Autodesk Inventor part; units mm, degrees
ref_plane "YZ Plane" through (0, 0, 0) normal (1, 0, 0) x (0, 1, 0)
ref_plane "XZ Plane" through (0, 0, 0) normal (0, 1, 0) x (-1, 0, 0)
ref_plane "XY Plane" through (0, 0, 0) normal (0, 0, 1) x (1, 0, 0)
sketch "Sketch1" plane through (0, 0, 0) normal (0, 1, 0) x (-1, 0, 0)
  line L0 (-2, 6.5) -> (2, 6.5)
  line L1 (2, 6.5) -> (2, -6.5)
  line L2 (2, -6.5) -> (-2, -6.5)
  line L3 (-2, -6.5) -> (-2, 6.5)
  line L4 (-2, 6.5) -> (2, -6.5) construction
  line L5 (2, 6.5) -> (-2, -6.5) construction
  point P0 (0, 0)
  dimension "d0" = 4
  dimension "d1" = 13
extrude "Extrusion1" add sketch "Sketch1" along normal blind 4
sketch "Sketch2" plane through (2, 0, 6.5) normal (1, 0, 0) x (0, 0, -1)
  line L0 (0, 0) -> (0, 4)
  line L1 (0, 2) -> (13, 2) construction
  line L2 (13, 0) -> (13, 4)
  line L3 (2, 0) -> (11, 0)
  line L4 (11, 4) -> (2, 4)
  arc A0 (2, 4) -> (2, 0) centre (2, 2) ccw
  arc A1 (11, 0) -> (11, 4) centre (11, 2) ccw
  line L5 (0, 4) -> (13, 4)
  line L6 (0, 0) -> (13, 0)
  point P0 (6.5, 0)
  point P1 (6.5, 2)
extrude "Extrusion2" cut sketch "Sketch2" against normal blind 2 contours L0 A0 L6 | L0 L5 A0 | A1 L2 L6 | L5 L2 A1
sketch "Sketch3" plane through (-2, 0, -6.5) normal (-1, 0, 0) x (0, 0, 1)
  arc A0 (2, 4) -> (0, 2) centre (2, 2) ccw
  line L0 (0, 0) -> (0, 4)
  line L1 (0, 4) -> (13, 4)
  arc A1 (0, 2) -> (2, 0) centre (2, 2) ccw
  arc A2 (2, 4) -> (2, 0) centre (2, 2) ccw
  line L2 (11, 4) -> (2, 4)
  arc A3 (11, 0) -> (11, 4) centre (11, 2) ccw
  line L3 (11, 0) -> (2, 0)
  line L4 (13, 0) -> (13, 4)
  line L5 (0, 0) -> (13, 0)
  point P0 (6.5, 0)
  point P1 (13, 2)
extrude "Extrusion3" cut sketch "Sketch3" against normal blind 1 contours A0 L0 L1 | A1 L5 L0 | L1 L4 A3 | L4 L5 A3
sketch "Sketch4" plane through (-2, 0, -4.5) normal (-1, 0, 0) x (0, 0, 1)
  arc A0 (0, 4) -> (-2, 2) centre (0, 2) ccw
  circle A1 centre (0, 2) radius 1.5
  arc A2 (11, 2) -> (9, 4) centre (9, 2) ccw
  circle A3 centre (9, 2) radius 1.5
  point P0 (4.5, 0)
  dimension "d8" = 3
  dimension "d9" = 3
mark "Mark1"
sketch "Sketch5" plane through (-2, 0, -4.5) normal (-1, 0, 0) x (0, 0, 1)
  circle A0 centre (3, 2) radius 1
  circle A1 centre (0, 2) radius 1.5
  circle A2 centre (9, 2) radius 1.5
  line L0 (0, 4) -> (9, 4)
  circle A3 centre (6, 2) radius 1
  point P0 (4.5, 0)
  dimension "d10" = 2
  dimension "d11" = 3
  dimension "d12" = 9
  dimension "d15" = 3
mark "Mark2"
sketch "Sketch6" plane through (-2, 2, -1.5) normal (-1, 0, 0) x (0, 0, 1)
  circle A0 centre (0, 0) radius 1
  circle A1 centre (0, 0) radius 0.5
  circle A2 centre (3, 0) radius 1
  circle A3 centre (3, 0) radius 0.5
  point P0 (1.5, -2)
  dimension "d20" = 1
  dimension "d21" = 1
extrude "Extrusion4" add sketch "Sketch6" along normal blind 2 contours A1 | A3
sketch "Sketch7" plane through (2, 0, 4.5) normal (1, 0, 0) x (0, 0, -1)
  circle A0 centre (0, 2) radius 1.5
  circle A1 centre (9, 2) radius 1.5
  point P0 (4.5, 0)
mark "Mark3"
sketch "Sketch8" plane through (2, 0, 4.5) normal (1, 0, 0) x (0, 0, -1)
  circle A0 centre (6, 2) radius 1
  circle A1 centre (3, 2) radius 1
  circle A2 centre (3, 2) radius 0.75
  circle A3 centre (6, 2) radius 0.75
  point P0 (4.5, 0)
  dimension "d24" = 1.5
  dimension "d25" = 1.5
mark "Mark4"
sketch "Sketch11" plane through (0, 0, 6.5) normal (1, 0, 0) x (0, 0, -1)
  line L0 (-2.865, 2) -> (15.865, 2) construction
  line L1 (-0.865, 0) -> (13.865, 0)
  line L2 (13.865, 4) -> (-0.865, 4)
  arc A0 (-0.865, 4) -> (-0.865, 0) centre (-0.865, 2) ccw
  arc A1 (13.865, 0) -> (13.865, 4) centre (13.865, 2) ccw
  line L3 (2, 0) -> (11, 0)
  point P0 (6.5, 0)
  point P1 (6.5, 2)
  point P2 (6.5, 4)
  point P3 (6.5, 0)
  dimension "d31" = 18.73
extrude "Extrusion7" add sketch "Sketch11" against normal blind 1
sketch "Sketch12" plane through (0, 0, 6.5) normal (1, 0, 0) x (0, 0, -1)
  arc A0 (-0.865, 4) -> (-0.865, 0) centre (-0.865, 2) ccw
  circle A1 centre (-1.6, 2) radius 0.75
  circle A2 centre (2, 2) radius 1.5
  point P0 (6.5, 0)
  dimension "d34" = 1.5
  dimension "d35" = 3.6
extrude "Extrusion8" cut sketch "Sketch12" against normal blind 1 contours A1
mirror "Mirror1" about plane through (0, 0, 0) normal (0, 0, 1) of "Extrusion8"
equation "\"d9\" = d8"
equation "\"d11\" = 0.333333 * d12"
equation "\"d15\" = d11"
equation "\"d21\" = d20"
equation "\"d25\" = d24"
properties part number "2_pin_ear_female"
Check sheet for the modelled part. Datum: model origin and axes. Units: mm. A direction names the side the tool comes from. Coordinates: 2 decimals unless noted, no trailing zeros. Order: outer loops, then holes, each group sorted by start corner. A loop starts at its lowest first (then second) coordinate and runs counter-clockwise, first axis right, second up. Notation, with made-up numbers: M 40,11.25 L 86,11.25 A28 cw 86,42.25 Z; hole C -20,-7 d11. An arc over 180 degrees is marked long. One line per question, with ' | ' between items. Start each with the question number.
Item 1: Sectioned sample at D-D on x = -3.5. Record the cut outline in (y, z), and give its area (3 significant figures).
Item 2: Access from +Z, -Z, +X, -X, +Y, -Y to the whole of each face (thin tool, end or side, straight path). Record for faces 5 (the cylindrical face through (-1.5, 2, -6.5)), 6 (the cylindrical face through (-1.5, 2, 6.5)), 7 (the cylindrical face through (1, 2, 6.5)), 8 (the cylindrical face through (-3, 2, 1)), 9 (the cylindrical face through (1, 2, -6.5)).
Item 3: Sectioned sample at A-A on y = 2. Record the cut outline in (x, z) (3 decimals).
Item 4: Mould release check, pull along Y, two halves, no side actions. Record for faces 1 (the cylindrical face through (-0.493, 2.225, 7.385)), 2 (the flat face through (2, 2, 0)), 3 (the flat face through (0, 4, 0)), 4 (the cylindrical face through (-0.493, 1.956, -9.365)): pulls with the +Y half, pulls with the -Y half, needs draft (parallel to the pull), parting line crosses it, or undercut.
Item 5: Material ranges on line 1 (X direction, y = 3.25, z = -3.75); line 2 (Y direction, x = -0.5, z = 8.1); line 3 (Z direction, x = -2.8, y = 1.75), recorded low to high.
Item 6: Gauge pin test, flat ends, axial feed: P1, Ø2, axis at y = 2.5, z = -7, coming from the -X side; P2, Ø1.5, axis at x = 1, y = 1, coming from the -Z side; P3, Ø2, axis at y = 2, z = 8.1, coming from the -X side; P4, Ø0.9, axis at y = 2, z = -8.1, coming from the -X side. Record the tip position at first contact, or that the pin passes through.
Item 7: Sectioned sample at C-C on z = 1.5. Record the cut outline in (x, y).
Item 8: Sectioned sample at B-B on z = -8. Record the cut outline in (x, y), and give its area (3 significant figures).
Answer below:
1) outline: C 2,-1.5 d1; C 2,1.5 d1 | area: 1.57 mm^2
2) face 5: -Z, -X | face 6: +Z, -X | face 7: +Z, +X | face 8: -X | face 9: -Z, +X
3) outline: M -4,-2 L -2,-2 L -2,-6.5 L -1,-6.5 L -1,-7.35 L 0,-7.35 L 0,-6.5 L 2,-6.5 L 2,6.5 L 0,6.5 L 0,7.35 L -1,7.35 L -1,6.5 L -2,6.5 L -2,2 L -4,2 L -4,1 L -2,1 L -2,-1 L -4,-1 Z; M -1,-9.365 L 0,-9.365 L 0,-8.85 L -1,-8.85 Z; M -1,8.85 L 0,8.85 L 0,9.365 L -1,9.365 Z
4) face 1: undercut | face 2: needs draft | face 3: pulls with the +Y half | face 4: parting line crosses it
5) line 1: x = -2 to 2 | line 2: y = 0.14 to 1.25, 2.75 to 3.86 | line 3: z = -1.93 to -1.07, 1.07 to 1.93
6) P1: stops at x = -2 | P2: stops at z = -6.48 | P3: stops at x = -1 | P4: passes through
7) outline: M -4,1.5 L -2,1.5 L -2,0 L 2,0 L 2,4 L -2,4 L -2,2.5 L -4,2.5 Z
8) outline: M -1,0.1 L 0,0.1 L 0,1.26 L -1,1.26 Z; M -1,2.74 L 0,2.74 L 0,3.9 L -1,3.9 Z | area: 2.31 mm^2
